For this review, use the dimensioned drawing (mm, ordinates from the lowest corner) and the shaded views. A direction names the side the tool comes from. Coordinates: 2 decimals unless noted, no trailing zeros. Write each loop counter-clockwise with the first axis right and the second up, starting at its lowest first coordinate (ties: lowest second). Pieces come first, ordered by that corner, then holes. Notation, with made-up numbers: M 59,31 L 63,31 A8 ccw 63,43 Z; hole C 87.25,-5 d10. An arc over 180 degrees is marked long. One line per question, with ' | ' between items.
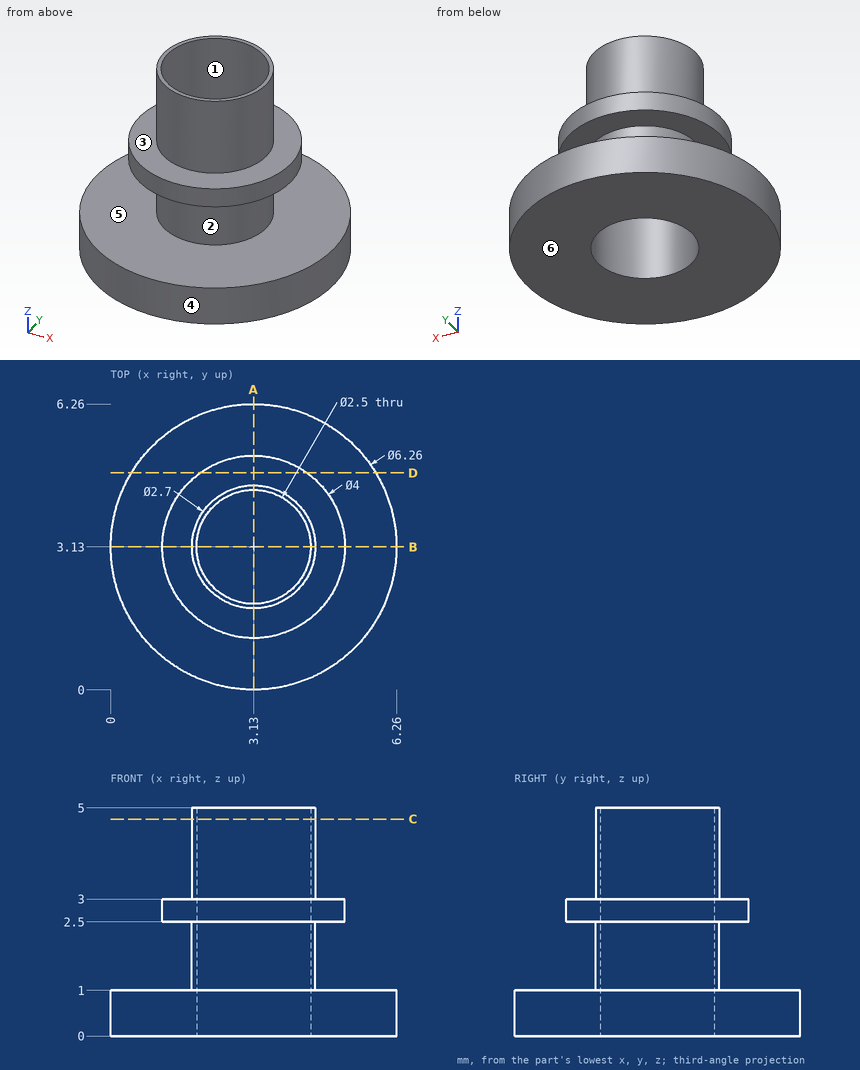
1) To check wall thickness, follow line 1 along Z through (x, y) = (5, 3.25); line 2 along Z through (x, y) = (5.25, 5.25); line 3 along X through (y, z) = (3.13, 2.6). State the ranges of each line that lie inside material, in increasing order. Write a range as [from, to].
Responses:
line 1: [0, 1], [2.5, 3] | line 2: [0, 1] | line 3: [1.13, 1.88], [4.38, 5.13]
2) Machinability: for the marked faces 1, 2 and 3, which of the approach directions +Z, -Z, +X, -X, +Y, -Y give a long, thin tool a straight path to every point of the face, cutting with its end or side? Answer none if there is none.
Responses:
face 1: +Z, -Z | face 2: none | face 3: +Z
3) We need section D-D on y = 4.75. State the section outline as (x, z) points.
Responses:
outline: M 0.45,0 L 5.81,0 L 5.81,1 L 0.45,1 Z; M 1.96,2.5 L 4.3,2.5 L 4.3,3 L 1.96,3 Z
4) We need section A-A on x = 3.13. State the section outline as (y, z) points, then the cut area to 3 significant figures.
Responses:
outline: M 0,0 L 1.88,0 L 1.88,5 L 1.78,5 L 1.78,3 L 1.13,3 L 1.13,2.5 L 1.78,2.5 L 1.78,1 L 0,1 Z; M 4.38,0 L 6.26,0 L 6.26,1 L 4.48,1 L 4.48,2.5 L 5.13,2.5 L 5.13,3 L 4.48,3 L 4.48,5 L 4.38,5 Z | area: 5.21 mm^2
5) The part is to be moulded in two halves that separate along Z. For the marked faces 4, 5 and 6, say which applies: +Z half, -Z half, draft (parallel to the pull), parting line (faces both ways), or undercut.
Responses:
face 4: draft | face 5: undercut | face 6: -Z half
6) We need section C-C on z = 4.75. State the section outline as (x, y) points.
Responses:
outline: C 3.13,3.13 d2.7; hole C 3.13,3.13 d2.5
7) Insertion check: pin 1 Ø1 at (x, y) = (4, 1) entering from +Z; pin 2 Ø1.5 at (x, y) = (3.13, 3.13) entering from -Z. Each pin has a flat end and moves straight along its axis. Give the tip position at first contact, or say it passes through.
Responses:
pin 1: z = 3 | pin 2: through
